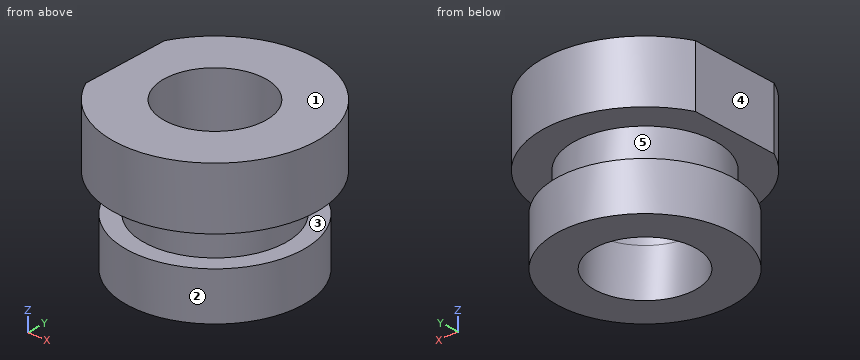
from build123d import *

# Parameters (mm, degrees)
F0_R     = 11
F0_R_2   = 7.9
F1_DEPTH = 9.5
F2_DEPTH = 5.8
F3_R     = 13.7
F3_R_2   = 11
F3_R_3   = 7.9
F4_DEPTH = 7.4


with BuildPart() as f1:
    # F0 (on Top) → F1 (new body)
    with BuildSketch(Plane.XY):
        with BuildLine():
            Line((-14.125, 7.0238878123), (-14.125, -7.0238878123))
            ThreePointArc((-14.125, -7.0238878123), (15.775, 0), (-14.125, 7.0238878123))
        make_face()
        Circle(F0_R, mode=Mode.SUBTRACT)
        Circle(F0_R)
        Circle(F0_R_2, mode=Mode.SUBTRACT)
    extrude(amount=F1_DEPTH)

    # F0 (on Top) → F2 (join)
    with BuildSketch(Plane.XY):
        Circle(F0_R)
        Circle(F0_R_2, mode=Mode.SUBTRACT)
    extrude(amount=-F2_DEPTH)

    # F3 (on face) → F4 (join)
    with BuildSketch(Plane(origin=(0, 0, -5.8), x_dir=(1, 0, 0), z_dir=(0, 0, -1))):
        Circle(F3_R)
        Circle(F3_R_2, mode=Mode.SUBTRACT)
        Circle(F3_R_2)
        Circle(F3_R_3, mode=Mode.SUBTRACT)
    extrude(amount=F4_DEPTH)


solid = f1.part
CAD build for the part. Positions are in the model's coordinates, mm. Face numbers are marked on the shaded views. A direction names the side the tool comes from. Coordinates: 2 decimals unless noted, no trailing zeros. Write each loop counter-clockwise with the first axis right and the second up, starting at its lowest first coordinate (ties: lowest second). Pieces come first, ordered by that corner, then holes. Notation, with made-up numbers: M 20,-18.5 L 43,-18.5 A20 cw 43,3.5 Z; hole C -32,72.25 d8. An arc over 180 degrees is marked long. Return JSON: item names as keys, results as strings.
Item 1: Drop flat-ended pins along their axis: pin 1 Ø5 at (x, z) = (3.5, -8) entering from +Y; pin 2 Ø1.5 at (x, z) = (-0.5, -2) entering from +Y; pin 3 Ø12 at (x, y) = (-0.5, 3.5) entering from +Z; pin 4 Ø5 at (x, z) = (-9.5, -5) entering from -Y. Give the stop position or say it passes through.
Findings below:
{"pin 1": "stops at y = 13.66", "pin 2": "stops at y = 11", "pin 3": "stops at z = 9.5", "pin 4": "stops at y = -11.7"}
Item 2: Slice it at B-B, the plane x = 0. Write the cut outline in (y, z) (3 decimals).
Findings below:
{"outline": "M -15.775,0 L -11,0 L -11,-5.8 L -13.7,-5.8 L -13.7,-13.2 L -7.9,-13.2 L -7.9,9.5 L -15.775,9.5 Z; M 7.9,-13.2 L 13.7,-13.2 L 13.7,-5.8 L 11,-5.8 L 11,0 L 15.775,0 L 15.775,9.5 L 7.9,9.5 Z"}
Item 3: Which spindle directions (+Z, -Z, +X, -X, +Y, -Y) get a long thin tool onto all of the face, cutting with end or side? Do the marked faces 4 and 5. Say none if no direction does.
Findings below:
{"face 4": "+Z, -Z, -X, +Y, -Y", "face 5": "none"}
Item 4: Probe line 1 (Z direction, x = -9.5, y = 9.5); line 2 (Y direction, x = 0, z = -2.6); line 3 (Y direction, x = 0, z = 4) (3 decimals). List the from-to ranges inside material, lowest first. Write a range as from..to.
Findings below:
{"line 1": "z = -13.2..-5.8, 0..9.5", "line 2": "y = -11..-7.9, 7.9..11", "line 3": "y = -15.775..-7.9, 7.9..15.775"}
Item 5: Two-plate mould, pull along Z, no slides. Class the marked faces 1, 2 and 3: +Z half, -Z half, draft (parallel to the pull), parting line (faces both ways), or undercut.
Findings below:
{"face 1": "+Z half", "face 2": "draft", "face 3": "undercut"}
Item 6: Slice it at C-C, the plane z = -3. Write the cut outline in (x, y), and give its area (3 significant figures).
Findings below:
{"outline": "C 0,0 d22; hole C 0,0 d15.8", "area": "184 mm2"}
Item 7: Slice it at A-A, the plane y = 0. Write the cut outline in (x, z) (3 decimals), and give its area (3 significant figures).
Findings below:
{"outline": "M -14.125,0 L -11,0 L -11,-5.8 L -13.7,-5.8 L -13.7,-13.2 L -7.9,-13.2 L -7.9,9.5 L -14.125,9.5 Z; M 7.9,-13.2 L 13.7,-13.2 L 13.7,-5.8 L 11,-5.8 L 11,0 L 15.775,0 L 15.775,9.5 L 7.9,9.5 Z", "area": "256 mm2"}
Item 8: Slice it at D-D, the plane x = 10.25. Write the cut outline in (y, z), and give its area (3 significant figures).
Findings below:
{"outline": "M -11.99,0 L -3.99,0 L -3.99,-5.8 L -9.09,-5.8 L -9.09,-13.2 L 9.09,-13.2 L 9.09,-5.8 L 3.99,-5.8 L 3.99,0 L 11.99,0 L 11.99,9.5 L -11.99,9.5 Z", "area": "409 mm2"}
